```python
from build123d import *

# Parameters (mm, degrees)
SKETCH1_W           = 228
SKETCH1_H           = 177
SKETCH1_W_2         = 90
SKETCH1_H_2         = 50
BOSS_EXTRUDE2_DEPTH = 200.582631371
CUT_EXTRUDE1_START  = -10
SKETCH2_W           = 108.838399528
SKETCH2_H           = 164.710968607
SKETCH2_W_2         = 60.282653626
SKETCH2_H_2         = 61.539971991
CUT_EXTRUDE1_DEPTH  = 180
SKETCH5_W           = 157.303446562
SKETCH5_H           = 179.645970641
CUT_EXTRUDE2_DEPTH  = 20


with BuildPart() as part:
    # Sketch1 → Boss-Extrude2 (new body)
    with BuildSketch(Plane(origin=(0, 0, 0), x_dir=(1, 0, 0), z_dir=(0, 1, 0))):
        Rectangle(SKETCH1_W, SKETCH1_H)
        with Locations((31, -2.231282948)):
            Rectangle(SKETCH1_W_2, SKETCH1_H_2, mode=Mode.SUBTRACT)
    extrude(amount=BOSS_EXTRUDE2_DEPTH)

    # Sketch2 → Cut-Extrude1 (cut)
    with BuildSketch(Plane(origin=(0, 200.582631371, 0), x_dir=(1, 0, 0), z_dir=(0, 1, 0)).offset(CUT_EXTRUDE1_START)):
        with Locations((-52.521027136, 0.352939873)):
            Rectangle(SKETCH2_W, SKETCH2_H)
        Polygon((109.79292582, 82.708424176), (1.898172628, 82.708424176), (1.898172628, 8.029391403), (62.180826254, 8.029391403), (109.79292582, 8.029391403), align=None)
        with Locations((32.039499441, -51.232558436)):
            Rectangle(SKETCH2_W_2, SKETCH2_H_2)
        Polygon((109.79292582, 8.029391403), (62.180826254, 8.029391403), (62.180826254, -20.46257244), (62.180826254, -82.002544431), (109.79292582, -82.002544431), align=None)
    extrude(amount=-CUT_EXTRUDE1_DEPTH, mode=Mode.SUBTRACT)

    # Sketch5 → Cut-Extrude2 (cut)
    with BuildSketch(Plane(origin=(114, 0, 0), x_dir=(0, 0, -1), z_dir=(1, 0, 0))):
        with Locations((0.425718885, 99.965893577)):
            Rectangle(SKETCH5_W, SKETCH5_H)
    extrude(amount=-CUT_EXTRUDE2_DEPTH, mode=Mode.SUBTRACT)


solid = part.part
```
Build history of the part. All positions in model axes, mm. A direction names the side the tool comes from. Round coordinates to 2 decimals unless told otherwise and drop trailing zeros. Write each loop counter-clockwise with the first axis right and the second up, starting at its lowest first coordinate (ties: lowest second). Pieces come first, ordered by that corner, then holes. Notation, with made-up numbers: (82.25, -20) - (102.25, -20) arc R22 ccw to (102.25, -3) - close; hole circle Ø10 at (28, 13). An arc over 180 degrees is marked (long way). Answer as CSV lines item,"result".
Q1. Cut at D-D (y = 50.5). Write the cut outline in (x, z).
Report:
outline,"(-114, -88.5) - (114, -88.5) - (114, -79.08) - (109.79, -79.08) - (109.79, -82.71) - (-106.94, -82.71) - (-106.94, 82) - (109.79, 82) - (109.79, 78.23) - (114, 78.23) - (114, 88.5) - (-114, 88.5) - close"
Q2. Tool access for faces 1 (the flat face through (30, 196, -22.769)), 2 (the flat face through (3, 102, -82.708)), 3 (the flat face through (-2, 99, 88.5)), 4 (the flat face through (112, 100, -79.077)): list every direction of +Z, -Z, +X, -X, +Y, -Y with a clear straight run to the whole face (end or side of a thin tool).
Report:
face 1,"+Y, -Y"
face 2,"none"
face 3,"+Z, +X, -X, +Y, -Y"
face 4,"+X"
Q3. Cut at C-C (x = -19.5). Write the cut outline in (y, z), and give its area (3 significant figures).
Report:
outline,"(0, -88.5) - (200.58, -88.5) - (200.58, 88.5) - (0, 88.5) - close; hole (10.58, -82.71) - (190.58, -82.71) - (190.58, 82) - (10.58, 82) - close"
area,"5,860 mm^2"
Q4. Drop a flat-ended pin along its axis: pin 1 (10 mm diameter, centred on y = 132, z = 19.5, fed in from +X). Give the stop position or say it passes through.
Report:
pin 1,"stops at x = -106.94"
Q5. Drill centre lines: probe 1 along Z at (x, y) = (-62, 94); probe 2 along X at (y, z) = (51, -80); probe 3 along Y at (x, z) = (-88.5, -30). Where is each one in solid material? Low to high. Write a range as [from, to].
Report:
probe 1,"z = [-88.5, -82.71], [82, 88.5]"
probe 2,"x = [-114, -106.94], [109.79, 114]"
probe 3,"y = [0, 10.58], [190.58, 200.58]"
Q6. Cut at A-A (z = -5.5). Write the cut outline in (x, y).
Report:
outline,"(-114, 0) - (-14, 0) - (-14, 10.58) - (-106.94, 10.58) - (-106.94, 190.58) - (-14, 190.58) - (-14, 200.58) - (-114, 200.58) - close; (76, 0) - (114, 0) - (114, 10.14) - (94, 10.14) - (94, 10.58) - (76, 10.58) - close; (76, 190.58) - (109.79, 190.58) - (109.79, 189.79) - (114, 189.79) - (114, 200.58) - (76, 200.58) - close"
Q7. Cut at B-B (x = 46). Write the cut outline in (y, z), and give its area (3 significant figures).
Report:
outline,"(0, -88.5) - (200.58, -88.5) - (200.58, -22.77) - (190.58, -22.77) - (190.58, -82.71) - (10.58, -82.71) - (10.58, -22.77) - (0, -22.77) - close; (0, 27.23) - (10.58, 27.23) - (10.58, 82) - (190.58, 82) - (190.58, 27.23) - (200.58, 27.23) - (200.58, 88.5) - (0, 88.5) - close"
area,"4,830 mm^2"
Q8. Pull direction X, two halves, no side cores. Call faces 5 (the flat face through (0, 102, 82.003)), 6 (the flat face through (-114, 99, 1)), 7 (the flat face through (114, 100, 79)), 8 (the flat face through (-27, 200.583, -1)): +X half, -X half, draft (parallel to the pull), parting line (faces both ways), or undercut.
Report:
face 5,"undercut"
face 6,"-X half"
face 7,"+X half"
face 8,"draft"
